from build123d import *

# Parameters (mm, degrees)
CUT_EXTRUDE1_DEPTH = 0.75
FILLET1_R          = 0.125


with BuildPart() as part:
    # Sketch1 → Revolve1 (revolve)
    with BuildSketch(Plane(origin=(0, 0, 0), x_dir=(0, 0, -1), z_dir=(1, 0, 0))):
        with BuildLine():
            Line((0, 1.5), (-1.5, 1.5))
            ThreePointArc((-1.5, 1.5), (-1.978515811, 0.925250119), (-2.3, 0.25))
            Line((-2.3, 0.25), (-2.155662433, 0))
            Line((-2.155662433, 0), (-1, 0))
            Line((-1, 0), (-1, -8))
            Line((-1, -8), (0, -8))
            Line((0, -8), (0, 1.5))
        make_face()
    revolve(axis=Axis((0, -8, 0), (0, 1, 0)))

    # Sketch2 → Cut-Extrude1 (cut)
    with BuildSketch(Plane(origin=(0, 1.5, 0), x_dir=(1, 0, 0), z_dir=(0, 1, 0))):
        Polygon((0, 1.154700538), (-1, 0.577350269), (-1, -0.577350269), (0, -1.154700538), (1, -0.577350269), (1, 0.577350269), align=None)
    extrude(amount=-CUT_EXTRUDE1_DEPTH, mode=Mode.SUBTRACT)

    # Fillet1
    fillet1_edges = [part.edges().sort_by_distance(p)[0] for p in [
        (0.5, 1.5, -0.866025404),
        (-0.5, 1.5, -0.866025404),
        (-1, 1.5, 0),
        (-0.5, 1.5, 0.866025404),
        (0.5, 1.5, 0.866025404),
        (1, 1.5, 0),
        (0, 1.5, -1.5),
    ]]
    fillet(fillet1_edges, radius=FILLET1_R)


solid = part.part
Verification items for the finished model (mm, model axes). Round coordinates to 2 decimals unless told otherwise and drop trailing zeros. Order: outer loops, then holes, each group sorted by start corner. A loop starts at its lowest first (then second) coordinate and runs counter-clockwise, first axis right, second up. Notation, with made-up numbers: (-37.5, -26) -> (-12.5, -26) arc R21 ccw to (-12.5, -14) -> close; hole circle Ø6 at (13.25, 7.5). An arc over 180 degrees is marked (long way). Put each result on its own line as item: value.
1) Depth check by flat-ended pin: pin 1 (1 mm diameter, centred on x = 0, z = 0.5, fed in from +Y); pin 2 (1.5 mm diameter, centred on y = -0.5, z = -1, fed in from -X); pin 3 (1.3 mm diameter, centred on x = 0.5, z = 1, fed in from -Y); pin 4 (0.7 mm diameter, centred on y = 1, z = 0, fed in from +X). Enter the tip coordinate at first touch or a pass-through.
Final values:
pin 1: stops at y = 0.75
pin 2: stops at x = -2.15
pin 3: stops at y = -8
pin 4: stops at x = 2.13
2) Mould release check, pull along X, two halves, no side actions. Record for faces 1 (the flat face through (0, 0.75, 0)), 2 (the flat face through (0, -8, 0)), 3 (the cylindrical face through (-1, -4, 0)): +X half, -X half, draft (parallel to the pull), parting line (faces both ways), or undercut.
Final values:
face 1: undercut
face 2: draft
face 3: parting line
3) Material ranges on line 1 (Y direction, x = -0.05, z = -0.45); line 2 (Z direction, x = -1.2, y = 1); line 3 (Z direction, x = 0.9, y = -2.5), recorded low to high.
Final values:
line 1: y = -8 to 0.75
line 2: z = -1.51 to 1.51
line 3: z = -0.44 to 0.44
4) Section check A-A (y = -2.75). Record the cut outline in (x, z), then the cut area to 3 significant figures.
Final values:
outline: circle Ø2 at (0, 0)
area: 3.14 mm^2
